```python
from build123d import *

# Parameters (mm, degrees)
F1_DEPTH = 50.8
F2_R     = 6.35
F3_DEPTH = 6.35
F4_R     = 12.7
F5_DEPTH = 19.05
F6_R     = 6.35
F7_DEPTH = 6.35


with BuildPart() as f1:
    # F0 (on Front) → F1 (new body)
    with BuildSketch(Plane.XZ):
        Polygon((0, 25.4), (0, 0), (25.4, 0), (558.8, 25.4), (584.2, 25.4), (584.2, 50.8), (558.8, 50.8), (25.4, 25.4), align=None)
    extrude(amount=F1_DEPTH)

    # F2 (on Top) → F3 (cut)
    with BuildSketch(Plane.XY):
        with Locations((12.7, -25.4)):
            Circle(F2_R)
    extrude(amount=F3_DEPTH, mode=Mode.SUBTRACT)

    # F4 (on Top) → F5 (cut)
    with BuildSketch(Plane.XY):
        with Locations((292.1, -25.4)):
            Circle(F4_R)
    extrude(amount=F5_DEPTH, mode=Mode.SUBTRACT)

    # F6 (on face) → F7 (cut)
    with BuildSketch(Plane(origin=(0, 0, 25.4), x_dir=(1, 0, 0), z_dir=(0, 0, -1))):
        with Locations((571.5, 25.4)):
            Circle(F6_R)
    extrude(amount=-F7_DEPTH, mode=Mode.SUBTRACT)


solid = f1.part
```
Model file for the job. Use its own axes, mm. A direction names the side the tool comes from. Give positions to 0.01 mm unless a question says otherwise; leave off trailing zeros. Write each loop counter-clockwise with the first axis right and the second up, starting at its lowest first coordinate (ties: lowest second). Pieces come first, ordered by that corner, then holes. Notation, with made-up numbers: (40.25, 0.5) - (55.25, 0.5) arc R19 cw to (55.25, 21.5) - close; hole circle Ø8 at (36, -29). An arc over 180 degrees is marked (long way). One line per question, with ' | ' between items. Start each with the question number.
(1) Pin check, flat tips, straight feed: P1, Ø11.5, axis at x = 571.5, y = -25.4, coming from the -Z side; P2, Ø12, axis at x = 458, y = -16, coming from the -Z side; P3, Ø20.5, axis at x = 574, y = -36.5, coming from the -Z side. Stop position of each tip, or through.
(2) Slice it at C-C on x = 154.5. Write the cut outline in (y, z).
(3) Slice it at A-A on x = 12.7. Write the cut outline in (y, z), plus the area to 3 significant figures.
(4) 3-axis set-ups, long thin cutter, end or side, ignore diameter. For faces 1 (the face through (574, -19, 25.4)), 2 (the face through (13, -25, 25.4)), 3 (the face through (571, -25, 31.75)): which of +Z, -Z, +X, -X, +Y, -Y reach the whole face in a straight line?
(5) Wall check: line 1 along Y through (x, z) = (292.1, 16.25); line 2 along Z through (x, y) = (269.5, -43.5); line 3 along Z through (x, y) = (403.5, -22.5). Give the ranges that are in metal, low to high. Write a range as from..to.
(6) Slice it at B-B on y = -7. Write the cut outline in (x, z), plus the area to 3 significant figures.
Results below:
1) P1: z = 31.75 | P2: z = 20.31 | P3: z = 25.4
2) outline: (-50.8, 6.15) - (0, 6.15) - (0, 31.55) - (-50.8, 31.55) - close
3) outline: (-50.8, 0) - (-31.75, 0) - (-31.75, 6.35) - (-19.05, 6.35) - (-19.05, 0) - (0, 0) - (0, 25.4) - (-50.8, 25.4) - close | area: 1,210 mm^2
4) face 1: -Z, +X, +Y, -Y | face 2: +Z, -X, +Y, -Y | face 3: -Z
5) line 1: -50.8..-38.1, -12.7..0 | line 2: 11.62..37.02 | line 3: 18..43.4
6) outline: (0, 0) - (25.4, 0) - (558.8, 25.4) - (584.2, 25.4) - (584.2, 50.8) - (558.8, 50.8) - (25.4, 25.4) - (0, 25.4) - close | area: 14,800 mm^2
